```python
from build123d import *

# Parameters (mm, degrees)
F2_R     = 5.08
F3_R     = 7.62
F4_R     = 14.2888037355
F5_DEPTH = 25.4


with BuildPart() as f1:
    # F0 (on Front) → F1 (revolve)
    with BuildSketch(Plane.XZ):
        with BuildLine():
            Line((0, 55.7674504817), (0, 0))
            Line((0, 0), (50.8806146681, 0))
            Line((50.8806146681, 0), (50.8806146681, 12.8399282694))
            Line((50.8806146681, 12.8399282694), (18.8766103238, 12.8399282694))
            Line((18.8766103238, 12.8399282694), (18.8766103238, 32.0040024817))
            add(Edge.make_bspline(
                [(18.8766103238, 32.0040024817), (21.8979616755, 34.2451012966), (31.0578233334, 44.0143150598), (19.2667769723, 55.8005396658), (18.8766103238, 55.7674504817)],
                knots=[0, 0, 0, 0, 0.4863492735, 0.9442337123, 0.9442337123, 0.9442337123, 0.9442337123], degree=3))
            Line((18.8766103238, 55.7674504817), (0, 55.7674504817))
        make_face()
    revolve(axis=Axis((0, 0, 27.8837252408), (0, 0, -1)))

    # F2
    f2_edges = [f1.edges().sort_by_distance(p)[0] for p in [
        (-18.87661, 0, 12.839928),
    ]]
    fillet(f2_edges, radius=F2_R)

    # F3
    f3_edges = [f1.edges().sort_by_distance(p)[0] for p in [
        (-50.880615, 0, 12.839928),
    ]]
    fillet(f3_edges, radius=F3_R)

    # F4 (on Top) → F5 (join)
    with BuildSketch(Plane.XY):
        Circle(F4_R)
    extrude(amount=F5_DEPTH)


solid = f1.part
```
Work out the finished part from the listing and answer in its coordinate system (mm). A direction names the side the tool comes from. Give positions to 0.01 mm unless a question says otherwise; leave off trailing zeros. Order: outer loops, then holes, each group sorted by start corner. A loop starts at its lowest first (then second) coordinate and runs counter-clockwise, first axis right, second up. Notation, with made-up numbers: (-6.5, 20.5) - (2.5, 20.5) arc R19 ccw to (2.5, 24.5) - close; hole circle Ø10 at (42.25, -10). An arc over 180 degrees is marked (long way). One line per item, written item: value. Start each with the question number.
1. Section A-A, the plane z = 21.5 is taken. Write down the section's boundary in (x, y), then the cut area to 3 significant figures.
2. Which of the six approach directions +Z, -Z, +X, -X, +Y, -Y give full straight-line access (tool end or side, diameter ignored) to faces 1 (the face through (-13.91, -12.76, 25.06)), 2 (the face through (0, 0, 55.767))?
3. Consider line 1 (Z direction, x = 18.5, y = -21); line 2 (Z direction, x = -14, y = -15); line 3 (Z direction, x = -21.5, y = 0). Determine where each line is inside the solid, lowest interval first.
4. Each of these flat-tipped pins is pushed along its axis until it touches: pin 1 Ø8 at (x, y) = (-26.5, -30.5) entering from -Z; pin 2 Ø4 at (y, z) = (-12.5, 23) entering from -X; pin 3 Ø2 at (y, z) = (-15, 36) entering from -X; pin 4 Ø5 at (y, z) = (12.5, 45.5) entering from -X. Where does it stop, or does it pass through?
Filled sheet:
1. outline: circle Ø37.75 at (0, 0)
1. area: 1,120 mm²
2. face 1: none
2. face 2: +Z, +X, -X, +Y, -Y
3. line 1: 0 to 12.84
3. line 2: 0 to 14.18, 33.37 to 54.27
3. line 3: 0 to 13.47, 34.33 to 53.14
4. pin 1: z = 0
4. pin 2: x = -15.69
4. pin 3: x = -18.6
4. pin 4: x = -23.72
